from build123d import *

# Parameters (mm, degrees)
SKETCH2_W           = 55
SKETCH2_H           = 55
BOSS_EXTRUDE1_DEPTH = 33.6
BOSS_EXTRUDE2_DEPTH = 3
SKETCH4_W           = 15
SKETCH4_H           = 15
SKETCH4_R           = 2.6
BOSS_EXTRUDE3_DEPTH = 9
CUT_EXTRUDE1_START  = -5
SKETCH6_R           = 4.4
SKETCH6_R_2         = 2.6
CUT_EXTRUDE1_DEPTH  = 5
CHAMFER1_SIZE       = 5
FILLET4_R           = 2
SKETCH7_W           = 24
SKETCH7_H           = 26.6
CUT_EXTRUDE2_DEPTH  = 67
SKETCH8_W           = 26.6
SKETCH8_H           = 16
CUT_EXTRUDE3_DEPTH  = 67
SKETCH11_W          = 12
SKETCH11_H          = 4
BOSS_EXTRUDE4_DEPTH = 5
SKETCH12_R          = 1.1
CUT_EXTRUDE5_DEPTH  = 4
FILLET8_R           = 2
SKETCH13_R          = 1.6
CUT_EXTRUDE6_DEPTH  = 10
CHAMFER2_SIZE       = 1


with BuildPart() as part:
    # Sketch2 → Boss-Extrude1 (new body)
    with BuildSketch(Plane.XY):
        with Locations((0, 0.476186899)):
            Rectangle(SKETCH2_W, SKETCH2_H)
        Polygon((21.118377871, -17.280631787), (21.118377871, 17.280631787), (17.280631787, 21.118377871), (-17.280631787, 21.118377871), (-21.118377871, 17.280631787), (-21.118377871, -17.280631787), (-17.280631787, -21.118377871), (17.280631787, -21.118377871), align=None, mode=Mode.SUBTRACT)
    extrude(amount=BOSS_EXTRUDE1_DEPTH)

    # Sketch3 → Boss-Extrude2 (add)
    with BuildSketch(Plane.XY.offset(33.6)):
        with BuildLine():
            Line((-7.954951288, 8.431138187), (-18.961411379, 19.437598278))
            Line((-18.961411379, 19.437598278), (-21.118377871, 17.280631787))
            Line((-21.118377871, 17.280631787), (-21.118377871, -17.280631787))
            Line((-21.118377871, -17.280631787), (-19.437598278, -18.961411379))
            Line((-19.437598278, -18.961411379), (-7.954951288, -7.478764389))
            ThreePointArc((-7.954951288, -7.478764389), (-11.25, 0.476186899), (-7.954951288, 8.431138187))
        make_face()
        with BuildLine():
            Line((-7.954951288, -7.478764389), (-19.437598278, -18.961411379))
            Line((-19.437598278, -18.961411379), (-17.280631787, -21.118377871))
            Line((-17.280631787, -21.118377871), (17.280631787, -21.118377871))
            Line((17.280631787, -21.118377871), (19.437598278, -18.961411379))
            Line((19.437598278, -18.961411379), (7.954951288, -7.478764389))
            ThreePointArc((7.954951288, -7.478764389), (0, -10.773813101), (-7.954951288, -7.478764389))
        make_face()
        with BuildLine():
            Line((21.118377871, 17.280631787), (18.961411379, 19.437598278))
            Line((18.961411379, 19.437598278), (7.954951288, 8.431138187))
            ThreePointArc((7.954951288, 8.431138187), (10.393644741, 4.781375513), (11.25, 0.476186899))
            ThreePointArc((11.25, 0.476186899), (10.393644741, -3.829001715), (7.954951288, -7.478764389))
            Line((7.954951288, -7.478764389), (19.437598278, -18.961411379))
            Line((19.437598278, -18.961411379), (21.118377871, -17.280631787))
            Line((21.118377871, -17.280631787), (21.118377871, 17.280631787))
        make_face()
        with BuildLine():
            Line((-17.280631787, 21.118377871), (-18.961411379, 19.437598278))
            Line((-18.961411379, 19.437598278), (-7.954951288, 8.431138187))
            ThreePointArc((-7.954951288, 8.431138187), (0, 11.726186899), (7.954951288, 8.431138187))
            Line((7.954951288, 8.431138187), (18.961411379, 19.437598278))
            Line((18.961411379, 19.437598278), (17.280631787, 21.118377871))
            Line((17.280631787, 21.118377871), (-17.280631787, 21.118377871))
        make_face()
        Polygon((-18.961411379, 19.437598278), (-27.5, 27.976186899), (-27.5, -27.023813101), (-19.437598278, -18.961411379), (-21.118377871, -17.280631787), (-21.118377871, 17.280631787), align=None)
        Polygon((-19.437598278, -18.961411379), (-27.5, -27.023813101), (27.5, -27.023813101), (19.437598278, -18.961411379), (17.280631787, -21.118377871), (-17.280631787, -21.118377871), align=None)
        Polygon((27.5, -27.023813101), (27.5, 27.976186899), (18.961411379, 19.437598278), (21.118377871, 17.280631787), (21.118377871, -17.280631787), (19.437598278, -18.961411379), align=None)
        Polygon((27.5, 27.976186899), (-27.5, 27.976186899), (-18.961411379, 19.437598278), (-17.280631787, 21.118377871), (17.280631787, 21.118377871), (18.961411379, 19.437598278), align=None)
    extrude(amount=BOSS_EXTRUDE2_DEPTH)

    # Sketch4 → Boss-Extrude3 (add)
    # profile 1 of 4: a face of its own
    with BuildSketch(Plane(origin=(0, 0, 0), x_dir=(-1, 0, 0), z_dir=(0, 0, -1))):
        with Locations((-35, 17.5)):
            Rectangle(SKETCH4_W, SKETCH4_H)
        with Locations((-35, 17.5)):
            Circle(SKETCH4_R, mode=Mode.SUBTRACT)
    # profile 2 of 4: a face of its own
    with BuildSketch(Plane(origin=(0, 0, 0), x_dir=(-1, 0, 0), z_dir=(0, 0, -1))):
        with Locations((35, 17.5)):
            Rectangle(SKETCH4_W, SKETCH4_H)
        with Locations((35, 17.5)):
            Circle(SKETCH4_R, mode=Mode.SUBTRACT)
    # profile 3 of 4: a face of its own
    with BuildSketch(Plane(origin=(0, 0, 0), x_dir=(-1, 0, 0), z_dir=(0, 0, -1))):
        with Locations((-35, -17.5)):
            Rectangle(SKETCH4_W, SKETCH4_H)
        with Locations((-35, -17.5)):
            Circle(SKETCH4_R, mode=Mode.SUBTRACT)
    # profile 4 of 4: a face of its own
    with BuildSketch(Plane(origin=(0, 0, 0), x_dir=(-1, 0, 0), z_dir=(0, 0, -1))):
        with Locations((17.5, -34.523813101)):
            Rectangle(SKETCH4_W, SKETCH4_H)
        with Locations((17.5, -34.523813101)):
            Circle(SKETCH4_R, mode=Mode.SUBTRACT)
    extrude(amount=-BOSS_EXTRUDE3_DEPTH)

    # Sketch6 → Cut-Extrude1 (cut)
    # profile 1 of 4: a face of its own
    with BuildSketch(Plane.XY.offset(9).offset(CUT_EXTRUDE1_START)):
        with Locations((-17.5, -34.523813101)):
            Circle(SKETCH6_R)
    # profile 2 of 4: a face of its own
    with BuildSketch(Plane.XY.offset(9).offset(CUT_EXTRUDE1_START)):
        with Locations((-35, 17.5)):
            Circle(SKETCH6_R)
    # profile 3 of 4: a face of its own
    with BuildSketch(Plane.XY.offset(9).offset(CUT_EXTRUDE1_START)):
        with Locations((35, -17.5)):
            Circle(SKETCH6_R)
        with Locations(Location((35, -17.5, 0), (0, 0, 180))):
            Circle(SKETCH6_R_2, mode=Mode.SUBTRACT)
    # profile 4 of 4: a face of its own
    with BuildSketch(Plane.XY.offset(9).offset(CUT_EXTRUDE1_START)):
        with Locations((35, 17.5)):
            Circle(SKETCH6_R)
    extrude(amount=CUT_EXTRUDE1_DEPTH, mode=Mode.SUBTRACT)

    # Chamfer1
    chamfer1_edges = [part.edges().sort_by_distance(p)[0] for p in [
        (27.5, -27.023813101, 18.3),
        (-27.5, -27.023813101, 18.3),
        (27.5, 27.976186899, 18.3),
        (-27.5, 27.976186899, 18.3),
    ]]
    chamfer(chamfer1_edges, length=CHAMFER1_SIZE)

    # Fillet4
    fillet4_edges = [part.edges().sort_by_distance(p)[0] for p in [
        (0, 27.976186899, 36.6),
        (27.5, 0.476186899, 36.6),
        (0, -27.023813101, 36.6),
        (-27.5, 0.476186899, 36.6),
        (-25, -42.023813101, 4.5),
        (-10, -42.023813101, 4.5),
        (-42.5, 10, 4.5),
        (-42.5, 25, 4.5),
        (42.5, -25, 4.5),
        (42.5, -10, 4.5),
        (42.5, 10, 4.5),
        (42.5, 25, 4.5),
    ]]
    fillet(fillet4_edges, radius=FILLET4_R)

    # Sketch7 → Cut-Extrude2 (cut)
    with BuildSketch(Plane.XZ.offset(27.023813101)):
        with Locations((2.5, 13.3)):
            Rectangle(SKETCH7_W, SKETCH7_H)
    extrude(amount=-CUT_EXTRUDE2_DEPTH, mode=Mode.SUBTRACT)

    # Sketch8 → Cut-Extrude3 (cut)
    with BuildSketch(Plane.ZY.offset(27.5)):
        with Locations((13.3, 0)):
            Rectangle(SKETCH8_W, SKETCH8_H)
    extrude(amount=-CUT_EXTRUDE3_DEPTH, mode=Mode.SUBTRACT)


with BuildPart() as body_2:
    # Mirror2: mirrored copy
    add(part.part.mirror(Plane(origin=(-25, -42.023813101, 9), x_dir=(0, 0, 1), z_dir=(0, 1, 0))))

    # Sketch11 → Boss-Extrude4 (add)
    with BuildSketch(Plane.ZY.offset(27.5)):
        with Locations((26, -65.023813101)):
            Rectangle(SKETCH11_W, SKETCH11_H)
    extrude(amount=BOSS_EXTRUDE4_DEPTH)

    # Sketch12 → Cut-Extrude5 (cut)
    with BuildSketch(Plane.XZ.offset(67.023813101)):
        with Locations(Location((-29.5, 29.5, 0), (0, 0, 270))):
            Circle(SKETCH12_R)
        with Locations(Location((-29.5, 23, 0), (0, 0, 270))):
            Circle(SKETCH12_R)
    extrude(amount=-CUT_EXTRUDE5_DEPTH, mode=Mode.SUBTRACT)

    # Fillet8
    fillet8_edges = [body_2.edges().sort_by_distance(p)[0] for p in [
        (-32.5, -65.023813101, 32),
        (-32.5, -65.023813101, 20),
    ]]
    fillet(fillet8_edges, radius=FILLET8_R)

    # Sketch13 → Cut-Extrude6 (cut)
    with BuildSketch(Plane.XY.offset(36.6)):
        with Locations((15.5, -100.023813101)):
            Circle(SKETCH13_R)
        with Locations((-15.5, -100.023813101)):
            Circle(SKETCH13_R)
        with Locations((-15.5, -69.023813101)):
            Circle(SKETCH13_R)
        with Locations((15.5, -69.023813101)):
            Circle(SKETCH13_R)
    extrude(amount=-CUT_EXTRUDE6_DEPTH, mode=Mode.SUBTRACT)

    # Chamfer2
    chamfer2_edges = [body_2.edges().sort_by_distance(p)[0] for p in [
        (13.9, -69.023813101, 36.6),
        (-17.1, -69.023813101, 36.6),
        (-17.1, -100.023813101, 36.6),
        (13.9, -100.023813101, 36.6),
    ]]
    chamfer(chamfer2_edges, length=CHAMFER2_SIZE)


solid = body_2.part
Read the model definition and answer for the solid it produces. Units are mm, in the model's axes. A direction names the side the tool comes from. Coordinates: 2 decimals unless noted, no trailing zeros. Order: outer loops, then holes, each group sorted by start corner. A loop starts at its lowest first (then second) coordinate and runs counter-clockwise, first axis right, second up. Notation, with made-up numbers: M 37,9 L 68,9 A23 cw 68,20 Z; hole C -5.75,57 d11. An arc over 180 degrees is marked long. Put each result on its own line as item: value. Start each with the question number.
Item 1: Section B-B, the plane z = 11.5 is taken. Count the separate pieces of the cut face and the enclosed holes in it, plus the area to 3 significant figures.
Item 2: Consider probe 1 along Y at (x, z) = (35, 6.2); probe 2 along Y at (x, z) = (35, 2.9); probe 3 along X at (y, z) = (-69, 20). Determine where each line is inside the solid, lowest interval first. Write a range as [from, to].
Item 3: Section A-A, the plane x = 35 is taken. Determine the outline of the cut face in (y, z), plus the area to 3 significant figures.
Item 4: For faces 5 (the face through (33, -59.048, 4)), 6 (the face through (2, -60, 26.6)), 7 (the face through (-42.5, -101, 4)), 8 (the face through (24, -92.048, 13)), 9 (the face through (19.226, -103.22, 16.565)), determine the directions among +Z, -Z, +X, -X, +Y, -Y from which every point of the face is accessible in a straight line to the end or side of a thin tool.
Item 5: Section D-D, the plane y = -89.5 is taken. Determine the outline of the cut face in (x, z), plus the area to 3 significant figures.
Item 6: Given pin 1 Ø2 at (x, z) = (-29.5, 23) entering from -Y; pin 2 Ø7 at (x, z) = (23.5, 10) entering from +Y; pin 3 Ø1 at (x, y) = (26.5, -64) entering from +Z; pin 4 Ø5.5 at (x, y) = (35, -66.55) entering from +Z, each flat-ended and moving along its own axis, determine where each tip first touches the part or whether it passes through.
Item 7: The mould has two halves that part along X. Classify faces 1 (the face through (-17, -42.024, 4)), 2 (the face through (-41.899, -108.477, 4.563)), 3 (the face through (-17.6, -46.7, 4)), 4 (the face through (15.292, -98.437, 34.614)): +X half, -X half, draft (parallel to the pull), parting line (faces both ways), or undercut.
Item 8: Section C-C, the plane x = 15.5 is taken. Determine the outline of the cut face in (y, z), plus the area to 3 significant figures.
Computed:
1. separate pieces: 4
1. enclosed holes: 0
1. area: 710 mm2
2. probe 1: y = [-109.05, -105.95], [-97.15, -94.05], [-74.05, -70.95], [-62.15, -59.05]
2. probe 2: y = [-109.05, -104.15], [-98.95, -94.05], [-74.05, -69.15], [-63.95, -59.05]
2. probe 3: x = [-27.5, -21.12], [21.12, 27.5]
3. outline: M -109.05,0 L -104.15,0 L -104.15,4 L -105.95,4 L -105.95,9 L -109.05,9 Z; M -98.95,0 L -94.05,0 L -94.05,9 L -97.15,9 L -97.15,4 L -98.95,4 Z; M -74.05,0 L -69.15,0 L -69.15,4 L -70.95,4 L -70.95,9 L -74.05,9 Z; M -63.95,0 L -59.05,0 L -59.05,9 L -62.15,9 L -62.15,4 L -63.95,4 Z
3. area: 140 mm2
4. face 5: +Z, -Z, +X, +Y
4. face 6: -Z, +Y, -Y
4. face 7: +Z, -Z, -X, +Y, -Y
4. face 8: -Z, +X, -X
4. face 9: -Z
5. outline: M -27.5,26.6 L -21.12,26.6 L -21.12,33.6 L -10.09,33.6 L -10.09,36.6 L -25.5,36.6 A2 ccw -27.5,34.6 Z; M 10.09,33.6 L 21.12,33.6 L 21.12,26.6 L 27.5,26.6 L 27.5,34.6 A2 ccw 25.5,36.6 L 10.09,36.6 Z
5. area: 192 mm2
6. pin 1: passes through
6. pin 2: stops at y = -57.02
6. pin 3: stops at z = 36.54
6. pin 4: stops at z = 4
7. face 1: draft
7. face 2: -X half
7. face 3: undercut
7. face 4: undercut
8. outline: M -112.02,0 L -105.17,0 L -105.17,33.6 L -101.62,33.6 L -101.62,35.6 L -102.62,36.6 L -110.02,36.6 A2 ccw -112.02,34.6 Z; M -98.42,33.6 L -70.62,33.6 L -70.62,35.6 L -71.62,36.6 L -97.42,36.6 L -98.42,35.6 Z; M -67.42,33.6 L -62.93,33.6 L -62.93,0 L -57.02,0 L -57.02,34.6 A2 ccw -59.02,36.6 L -66.42,36.6 L -67.42,35.6 Z
8. area: 571 mm2
